Geometry: see drawing. Coordinates: mm, zero at the bounding-box minimum. Coordinates: 2 decimals unless noted, no trailing zeros. Order: outer loops, then holes, each group sorted by start corner. A loop starts at its lowest first (then second) coordinate and runs counter-clockwise, first axis right, second up. Notation, with made-up numbers: M 54.25,55.25 L 87.25,55.25 A37 cw 87.25,93.25 Z; hole C 89.25,80.5 d6. An arc over 180 degrees is marked long. One line per item, written item: value.
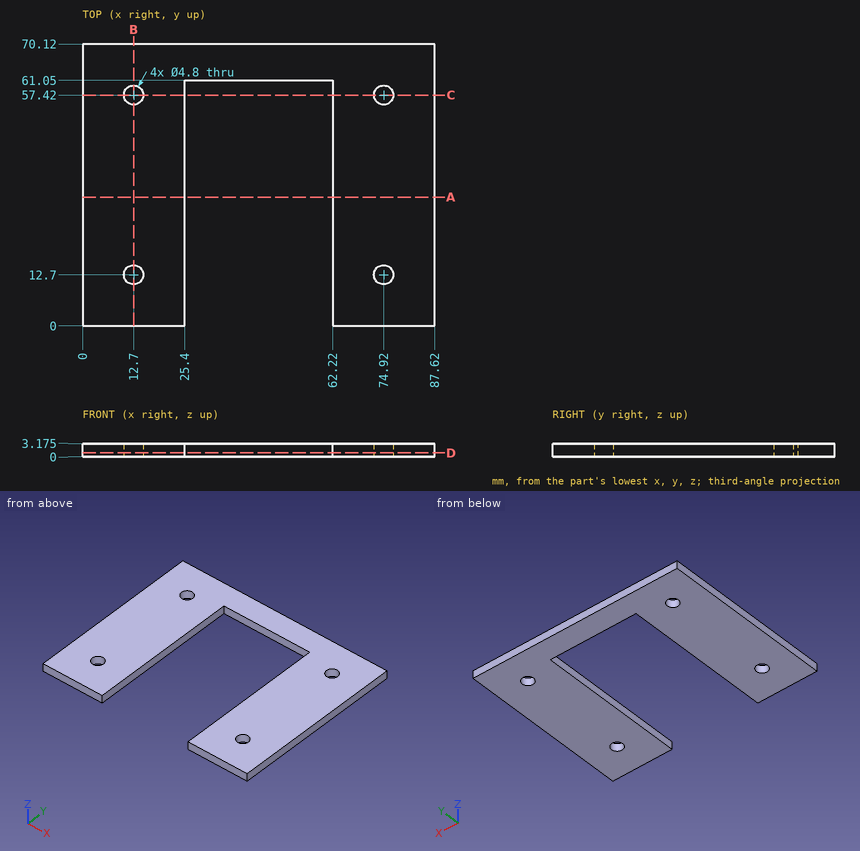
(1) Cut plane C-C on y = 57.42. Output: boundary loops of the cut face in (x, z) (1 decimal), plus the area to 3 significant figures.
Data:
outline: M 0,0 L 10.3,0 L 10.3,3.2 L 0,3.2 Z; M 15.1,0 L 25.4,0 L 25.4,3.2 L 15.1,3.2 Z; M 62.2,0 L 72.5,0 L 72.5,3.2 L 62.2,3.2 Z; M 77.3,0 L 87.6,0 L 87.6,3.2 L 77.3,3.2 Z
area: 131 mm2
(2) First-contact query: pin 1 (12 mm diameter, centred on x = 32, y = 15.5, fed in from -Z); pin 2 (1 mm diameter, centred on x = 40.5, z = 2, fed in from -Y). Flat tips, straight axial feed; report the tip coordinate or a pass-through.
Data:
pin 1: passes through
pin 2: stops at y = 61.05
(3) Ray query, line 1 (Y direction, x = 12.7, z = 2.2); line 2 (Y direction, x = 75.5, z = 2.45); line 3 (X direction, y = 23, z = 0.9). Return the intervals inside material, ascending. Write a range as from..to.
Data:
line 1: y = 0..10.3, 15.1..55.02, 59.82..70.12
line 2: y = 0..10.37, 15.03..55.09, 59.75..70.12
line 3: x = 0..25.4, 62.22..87.62
(4) Cut plane B-B on x = 12.7. Output: boundary loops of the cut face in (y, z) (1 decimal).
Data:
outline: M 0,0 L 10.3,0 L 10.3,3.2 L 0,3.2 Z; M 15.1,0 L 55,0 L 55,3.2 L 15.1,3.2 Z; M 59.8,0 L 70.1,0 L 70.1,3.2 L 59.8,3.2 Z
(5) Cut plane A-A on y = 32. Output: boundary loops of the cut face in (x, z) (1 decimal).
Data:
outline: M 0,0 L 25.4,0 L 25.4,3.2 L 0,3.2 Z; M 62.2,0 L 87.6,0 L 87.6,3.2 L 62.2,3.2 Z
(6) Cut plane D-D on z = 0.9. Output: boundary loops of the cut face in (x, y), plus the area to 3 significant figures.
Data:
outline: M 0,0 L 25.4,0 L 25.4,61.05 L 62.22,61.05 L 62.22,0 L 87.62,0 L 87.62,70.12 L 0,70.12 Z; hole C 12.7,12.7 d4.8; hole C 12.7,57.42 d4.8; hole C 74.92,12.7 d4.8; hole C 74.92,57.42 d4.8
area: 3,820 mm2
